Check sheet for the modelled part. Datum: model origin and axes. Units: mm. A direction names the side the tool comes from. Give positions to 0.01 mm unless a question says otherwise; leave off trailing zeros. Write each loop counter-clockwise with the first axis right and the second up, starting at its lowest first coordinate (ties: lowest second). Pieces come first, ordered by that corner, then holes. Notation, with made-up numbers: (1, 14) -> (50, 14) arc R38 ccw to (50, 52) -> close; hole circle Ø8 at (82, -0.5). An arc over 180 degrees is marked (long way). Use a Markdown table: item, result. Add a question column.
1. Release check for a two-part mould opening along Z. For faces 1 (the flat face through (56.902, 27.905, -51.333)), 2 (the flat face through (50, 6, -101.6)), 3 (the flat face through (50, 12.7, -97)) record: released by +Z, released by -Z, zero draft, split by the parting line, or undercut.
2. Cross-section at B-B (y = 5). Enter the section's corners in (x, z).
3. Set-up check for faces 4 (the flat face through (34.342, 63.146, -30.837)), 5 (the flat face through (101.6, 6, -50)): record each of +Z, -Z, +X, -X, +Y, -Y from which the full face is reachable in a straight line by a thin tool's end or side.
4. Gauge pin test, flat ends, axial feed: P1, Ø1.5, axis at y = 11.5, z = -44, coming from the +X side; P2, Ø3, axis at y = 32, z = -87.5, coming from the -X side; P3, Ø1.5, axis at x = 63, z = -35.5, coming from the +Y side. Record the tip position at first contact, or that the pin passes through.
5. Cross-section at A-A (z = -24). Enter the section's corners in (x, y).
6. Scan lines: probe 1 along Y at (x, z) = (91, -7.5); probe 2 along Z at (x, y) = (64.5, 40); probe 3 along Z at (x, y) = (40, 40.5). Record each from-to range of solid material in increasing order. Write a range as [from, to].
from build123d import *

# Parameters (mm, degrees)
SKETCH1_W           = 101.6
SKETCH1_H           = 101.6
BOSS_EXTRUDE1_DEPTH = 12.7
SKETCH4_R           = 44.45
SKETCH4_R_2         = 38.1
BOSS_EXTRUDE5_DEPTH = 1
BOSS_EXTRUDE6_REACH = 141.847
SKETCH7_R           = 44.45
SKETCH8_R           = 44.45
SKETCH8_R_2         = 38.1
BOSS_EXTRUDE7_DEPTH = 24.4


with BuildPart() as part:
    # Sketch1 → Boss-Extrude1 (new body)
    with BuildSketch(Plane(origin=(0, 0, 0), x_dir=(1, 0, 0), z_dir=(0, 1, 0))):
        with Locations((50.8, 50.8)):
            Rectangle(SKETCH1_W, SKETCH1_H)
    extrude(amount=BOSS_EXTRUDE1_DEPTH)

    # Boss-Extrude6: up to this face of the body (flat: up to its plane)
    boss_extrude6_end = Plane(part.part.faces().sort_by_distance((50.8, 12.7, -50.8))[0])
    # Sketch7 → Boss-Extrude6 (add, up to the picked face)
    with BuildSketch(Plane(origin=(15.624623468, 42.928300165, 0), x_dir=(0.9396926207859082, -0.34202014332566943, 0), z_dir=(-0.34202014332566943, -0.9396926207859082, 0)), mode=Mode.PRIVATE) as boss_extrude6_sk1:
        with Locations(Location((43.392729316, -50.8, 0), (0, 0, 180))):
            Circle(SKETCH7_R)
    boss_extrude6_tool1 = split(extrude(boss_extrude6_sk1.sketch, amount=BOSS_EXTRUDE6_REACH, mode=Mode.PRIVATE), bisect_by=boss_extrude6_end, keep=Keep.BOTH, mode=Mode.PRIVATE)


with BuildPart() as body_2:
    # Sketch4 → Boss-Extrude5 (new body)
    with BuildSketch(Plane(origin=(15.966643611, 43.867992786, 0), x_dir=(0, 0, -1), z_dir=(0.34202014332566943, 0.9396926207859081, 0))):
        with Locations(Location((50.8, -43.392729316, 0), (0, 0, 90))):
            Circle(SKETCH4_R)
        with Locations(Location((50.8, -43.392729316, 0), (0, 0, 90))):
            Circle(SKETCH4_R_2, mode=Mode.SUBTRACT)
    extrude(amount=-BOSS_EXTRUDE5_DEPTH)


with BuildPart() as part_1:
    add(part.part)

    add(body_2.part)  # Boss-Extrude6 merges body 2
    add(boss_extrude6_tool1.solids().sort_by(Axis((56.400451, 28.087113, -50.8), (-0.34202014332566943, -0.9396926207859082, 0)))[0])

    # Sketch8 → Boss-Extrude7 (add)
    with BuildSketch(Plane(origin=(15.966643611, 43.867992786, 0), x_dir=(0.9396926207859082, -0.34202014332566943, 0), z_dir=(0.34202014332566943, 0.9396926207859082, 0))):
        with Locations(Location((43.392729316, 50.8, 0), (0, 0, 180))):
            Circle(SKETCH8_R)
        with Locations(Location((43.392729316, 50.8, 0), (0, 0, 180))):
            Circle(SKETCH8_R_2, mode=Mode.SUBTRACT)
    extrude(amount=BOSS_EXTRUDE7_DEPTH)


solid = part_1.part
Worked answers:
| question | item | result |
|---|---|---|
| 1 | face 1 | undercut |
| 1 | face 2 | released by -Z |
| 1 | face 3 | zero draft |
| 2 | outline | (0, -101.6) -> (101.6, -101.6) -> (101.6, 0) -> (0, 0) -> close |
| 3 | face 4 | +Z, -Z, +X, +Y |
| 3 | face 5 | +Z, -Z, +X, -Y |
| 4 | P1 | stops at x = 101.6 |
| 4 | P2 | stops at x = 28.87 |
| 4 | P3 | stops at y = 25.96 |
| 5 | outline | (0, 0) -> (101.6, 0) -> (101.6, 12.7) -> (88.54, 12.7) -> (98.41, 39.83) -> (90.54, 42.69) -> (81.85, 18.82) -> (30.95, 37.35) -> (39.64, 61.22) -> (31.76, 64.08) -> (13.06, 12.7) -> (0, 12.7) -> close |
| 6 | probe 1 | y = [0, 12.7] |
| 6 | probe 2 | z = [-95.11, -88.74], [-12.86, -6.49] |
| 6 | probe 3 | z = [-90.67, -83.44], [-18.16, -10.93] |
